```python
from build123d import *

# Parameters (mm, degrees)
BOSS_EXTRUDE1_DEPTH = 100
CUT_EXTRUDE2_DEPTH  = 20
CUT_EXTRUDE3_START  = -20
CUT_EXTRUDE3_DEPTH  = 20
SKETCH10_R          = 40
BOSS_EXTRUDE6_DEPTH = 20
BOSS_EXTRUDE7_START = 20
SKETCH11_R          = 40
BOSS_EXTRUDE7_DEPTH = 20
SKETCH19_R          = 40
CUT_EXTRUDE7_DEPTH  = 285
SKETCH16_W          = 60
SKETCH16_H          = 150
CUT_EXTRUDE8_DEPTH  = 285


with BuildPart() as part:
    # Sketch1 → Boss-Extrude1 (new body)
    with BuildSketch(Plane(origin=(0, 0, 0), x_dir=(0, 0, -1), z_dir=(1, 0, 0))):
        with BuildLine():
            Line((-74.767803634, 0), (-74.767803634, 600))
            ThreePointArc((-74.767803634, 600), (0, 674.767803634), (74.767803634, 600))
            Line((74.767803634, 600), (74.767803634, 0))
            ThreePointArc((74.767803634, 0), (0, -74.767803634), (-74.767803634, 0))
        make_face()
    extrude(amount=BOSS_EXTRUDE1_DEPTH)

    # Sketch8 → Cut-Extrude2 (cut)
    with BuildSketch(Plane.ZY):
        with BuildLine():
            Line((-74.767803634, 600), (-74.767803634, 525))
            Line((-74.767803634, 525), (74.767803634, 525))
            Line((74.767803634, 525), (74.767803634, 600))
            ThreePointArc((74.767803634, 600), (0, 674.767803634), (-74.767803634, 600))
        make_face()
    extrude(amount=-CUT_EXTRUDE2_DEPTH, mode=Mode.SUBTRACT)

    # Sketch7 → Cut-Extrude3 (cut)
    with BuildSketch(Plane(origin=(100, 0, 0), x_dir=(0, 0, -1), z_dir=(1, 0, 0)).offset(CUT_EXTRUDE3_START)):
        with BuildLine():
            Line((-74.767803634, 600), (-74.767803634, 525))
            Line((-74.767803634, 525), (74.767803634, 525))
            Line((74.767803634, 525), (74.767803634, 600))
            ThreePointArc((74.767803634, 600), (0, 674.767803634), (-74.767803634, 600))
        make_face()
    extrude(amount=CUT_EXTRUDE3_DEPTH, mode=Mode.SUBTRACT)

    # Sketch10 → Boss-Extrude6 (add)
    with BuildSketch(Plane(origin=(80, 0, 0), x_dir=(0, 0, -1), z_dir=(1, 0, 0))):
        with Locations(Location((0, 600, 0), (0, 0, 180))):
            Circle(SKETCH10_R)
    extrude(amount=BOSS_EXTRUDE6_DEPTH)

    # Sketch11 → Boss-Extrude7 (add)
    with BuildSketch(Plane.ZY.offset(-20).offset(BOSS_EXTRUDE7_START)):
        with Locations((0, 600)):
            Circle(SKETCH11_R)
    extrude(amount=-BOSS_EXTRUDE7_DEPTH)

    # Sketch19 → Cut-Extrude7 (cut)
    with BuildSketch(Plane.ZY):
        Circle(SKETCH19_R)
    extrude(amount=-CUT_EXTRUDE7_DEPTH, mode=Mode.SUBTRACT)

    # Sketch16 → Cut-Extrude8 (cut)
    with BuildSketch(Plane.XY.offset(74.767803634)):
        with Locations((50, 0)):
            Rectangle(SKETCH16_W, SKETCH16_H)
    extrude(amount=-CUT_EXTRUDE8_DEPTH, mode=Mode.SUBTRACT)


solid = part.part
```
Source: CAD feature listing. Evaluate the final solid. Frame: model axes, mm. A direction names the side the tool comes from. Round coordinates to 2 decimals unless told otherwise and drop trailing zeros. Write each loop counter-clockwise with the first axis right and the second up, starting at its lowest first coordinate (ties: lowest second). Pieces come first, ordered by that corner, then holes. Notation, with made-up numbers: M 34,-29 L 73,-29 A6 ccw 73,-18 Z; hole C 68.5,50 d1. An arc over 180 degrees is marked long. Use CSV: the item, a comma, the result in double quotes. Start each with the question number.
Q1. Line query: line 1 (Y direction, x = 8, z = 0); line 2 (Y direction, x = 85.5, z = -11); line 3 (X direction, y = -42, z = 26). Output: solid intervals per line, ascending. Write a range as from..to.
Q2. Access query for faces 5 (the face through (10, 525, -1)), 6 (the face through (9.86, 560.95, -8.67)), 7 (the face through (80, 32, -32)), 8 (the face through (89.86, 639.05, -8.67)). Directions: +Z, -Z, +X, -X, +Y, -Y. A direction counts if a zero-diameter tool reaches every point of the face in a straight line with its end or side. Return the directions, or none.
Q3. Pull-direction query (X, two-part tool) for faces 1 (the face through (20, 32, -32)), 2 (the face through (0, 229, -1)), 3 (the face through (9.86, -74.75, -1.64)), 4 (the face through (80, 568, -32)); classes: +X half, -X half, draft (parallel to the pull), parting line (faces both ways), or undercut.
Q4. Cut plane C-C on y = 60.5. Output: boundary loops of the cut face in (x, z), plus the area to 3 significant figures.
Q5. Cut plane A-A on x = 7. Output: boundary loops of the cut face in (y, z).
Q6. First-contact query: P1, Ø10, axis at x = 38.5, z = -0.5, coming from the -Y side; P2, Ø10, axis at x = 11.5, z = -27.5, coming from the +Y side; P3, Ø8, axis at y = 149.5, z = -19, coming from the -X side; P4, Ø10, axis at x = 95, z = 14.5, coming from the +Y side. Flat tips, straight axial feed; report the tip coordinate or a pass-through.
Q7. Cut plane B-B on z = 0. Output: boundary loops of the cut face in (x, y).
Q8. Cut plane D-D on z = 29.5. Output: boundary loops of the cut face in (x, y), plus the area to 3 significant figures.
Results found:
1,line 1,"-74.77..-40, 40..525, 560..640"
1,line 2,"-73.95..-38.46, 38.46..525, 561.54..638.46"
1,line 3,"0..20, 80..100"
2,face 5,"+Z, -Z, -X"
2,face 6,"-X"
2,face 7,"+Z, -Z, -Y"
2,face 8,"+X"
3,face 1,"undercut"
3,face 2,"-X half"
3,face 3,"draft"
3,face 4,"+X half"
4,outline,"M 0,-74.77 L 20,-74.77 L 20,74.77 L 0,74.77 Z; M 80,-74.77 L 100,-74.77 L 100,74.77 L 80,74.77 Z"
4,area,"5,980 mm^2"
5,outline,"M 0,-74.77 L 525,-74.77 L 525,74.77 L 0,74.77 A74.77 ccw Z; C 600,0 d80; hole C 0,0 d80"
6,P1,"y = 75"
6,P2,"y = 633.07"
6,P3,"x = 0"
6,P4,"y = 638.86"
7,outline,"M 0,-74.77 L 20,-74.77 L 20,-40 L 0,-40 Z; M 0,40 L 20,40 L 20,75 L 80,75 L 80,40 L 100,40 L 100,525 L 80,525 L 80,560 L 100,560 L 100,640 L 80,640 L 80,674.77 L 20,674.77 L 20,640 L 0,640 L 0,560 L 20,560 L 20,525 L 0,525 Z; M 80,-74.77 L 100,-74.77 L 100,-40 L 80,-40 Z"
8,outline,"M 0,-68.7 L 20,-68.7 L 20,-27.01 L 0,-27.01 Z; M 0,27.01 L 20,27.01 L 20,75 L 80,75 L 80,27.01 L 100,27.01 L 100,525 L 80,525 L 80,572.99 L 100,572.99 L 100,627.01 L 80,627.01 L 80,668.7 L 20,668.7 L 20,627.01 L 0,627.01 L 0,572.99 L 20,572.99 L 20,525 L 0,525 Z; M 80,-68.7 L 100,-68.7 L 100,-27.01 L 80,-27.01 Z"
8,area,"59,400 mm^2"
